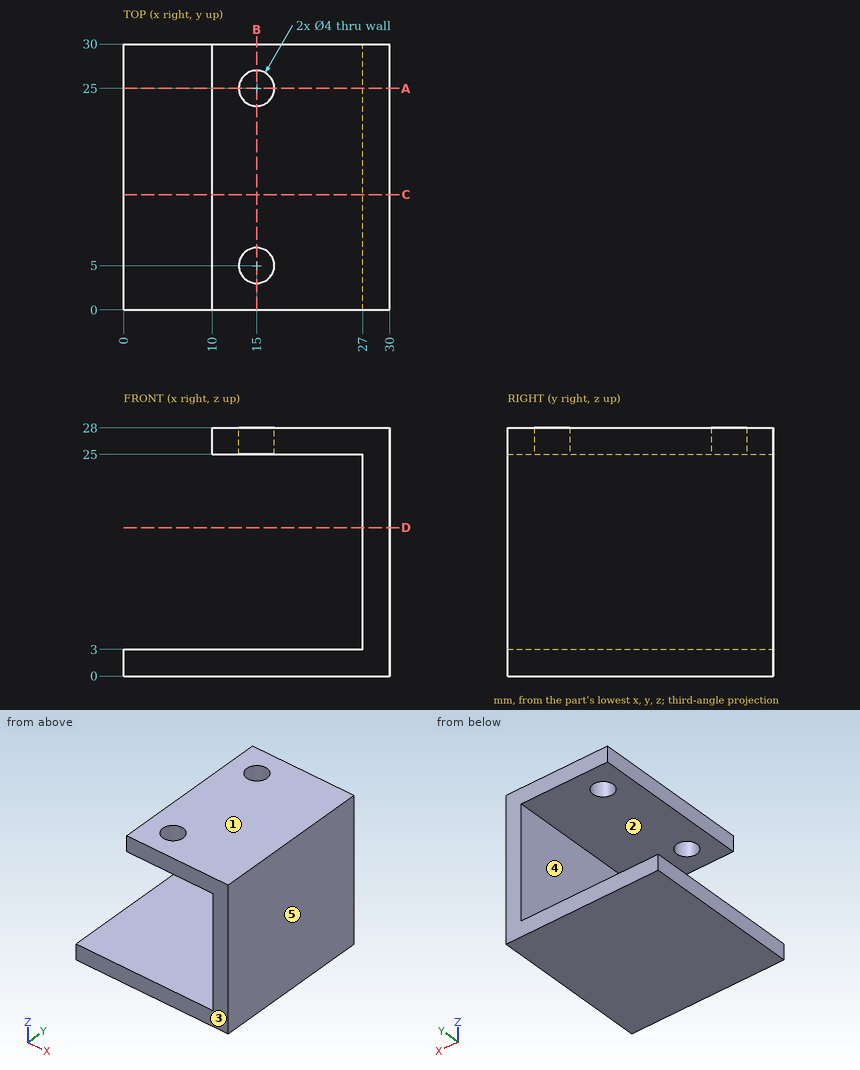
Answer from the drawing. Dimensions are ordinates in mm from the lowest x, y and z of the part. A direction names the side the tool comes from. Give positions to 0.01 mm unless a question says otherwise; leave off trailing zeros. Order: outer loops, then holes, each group sorted by start corner. A loop starts at its lowest first (then second) coordinate and runs counter-clockwise, first axis right, second up. Notation, with made-up numbers: (89, 31.5) - (99, 31.5) arc R38 ccw to (99, 70.5) - close; hole circle Ø6 at (13.5, -28.5). An arc over 180 degrees is marked (long way). One line per item, written item: value. Start each with the question number.
1) Given pin 1 Ø8.5 at (x, y) = (14.5, 11.5) entering from -Z; pin 2 Ø2 at (y, z) = (25, 12.5) entering from -X; pin 3 Ø1.5 at (y, z) = (19, 26.5) entering from -X, each flat-ended and moving along its own axis, determine where each tip first touches the part or whether it passes through.
2) A cutting plane is placed at C-C on y = 13. Give the vertices of the cut face in (x, z).
3) Find the intervals of material crossed by L1, parallel to Y at x = 15, z = 26.9; L2, parallel to X at y = 5, z = 27.2; L3, parallel to Z at x = 1.75, y = 2.75, in increasing order.
4) The mould has two halves that part along Z. Classify the marked faces 1, 2 and 3: released by +Z, released by -Z, zero draft, split by the parting line, or undercut.
5) A cutting plane is placed at B-B on x = 15. Give the vertices of the cut face in (y, z), then the cut area to 3 significant figures.
6) A cutting plane is placed at A-A on y = 25. Give the vertices of the cut face in (x, z).
7) A cutting plane is placed at D-D on z = 16.75. Give the vertices of the cut face in (x, y), then the cut area to 3 significant figures.
8) A tool of negligible diameter and unlimited length cuts with its end or side. For the marked faces 4 and 5, from which of +Z, -Z, +X, -X, +Y, -Y can it reach the whole face along a straight path? Write none if from no direction.
Answer sheet:
1. pin 1: stops at z = 0
1. pin 2: stops at x = 27
1. pin 3: stops at x = 10
2. outline: (0, 0) - (30, 0) - (30, 28) - (10, 28) - (10, 25) - (27, 25) - (27, 3) - (0, 3) - close
3. L1: y = 0 to 3, 7 to 23, 27 to 30
3. L2: x = 10 to 13, 17 to 30
3. L3: z = 0 to 3
4. face 1: released by +Z
4. face 2: undercut
4. face 3: zero draft
5. outline: (0, 0) - (30, 0) - (30, 3) - (0, 3) - close; (0, 25) - (3, 25) - (3, 28) - (0, 28) - close; (7, 25) - (23, 25) - (23, 28) - (7, 28) - close; (27, 25) - (30, 25) - (30, 28) - (27, 28) - close
5. area: 156 mm2
6. outline: (0, 0) - (30, 0) - (30, 28) - (17, 28) - (17, 25) - (27, 25) - (27, 3) - (0, 3) - close; (10, 25) - (13, 25) - (13, 28) - (10, 28) - close
7. outline: (27, 0) - (30, 0) - (30, 30) - (27, 30) - close
7. area: 90.0 mm2
8. face 4: -X, +Y, -Y
8. face 5: +Z, -Z, +X, +Y, -Y
